Check sheet for the modelled part. Datum: model origin and axes. Units: mm. A direction names the side the tool comes from. Round coordinates to 2 decimals unless told otherwise and drop trailing zeros. Write each loop counter-clockwise with the first axis right and the second up, starting at its lowest first coordinate (ties: lowest second). Pieces come first, ordered by that corner, then holes.
from build123d import *

# Parameters (mm, degrees)
SKETCH1_W           = 60
SKETCH1_H           = 40
BOSS_EXTRUDE1_DEPTH = 4
CHAMFER1_SIZE       = 3
SKETCH2_W           = 36
SKETCH2_H           = 24
CUT_EXTRUDE1_DEPTH  = 1.5
SKETCH3_W           = 4
SKETCH3_H           = 24
BOSS_EXTRUDE2_DEPTH = 23
CHAMFER2_SIZE       = 3
CHAMFER3_SIZE       = 2
CHAMFER4_SIZE       = 2
CHAMFER5_SIZE       = 2
CUT_EXTRUDE2_DEPTH  = 2.5
SKETCH7_R           = 2.604037506
CUT_EXTRUDE3_DEPTH  = 70.285640648
CUT_EXTRUDE4_DEPTH  = 2.5
SKETCH12_R          = 2.604037506
CUT_EXTRUDE6_DEPTH  = 68.485183559


with BuildPart() as part:
    # Sketch1 → Boss-Extrude1 (new body)
    with BuildSketch(Plane(origin=(0, 0, 0), x_dir=(1, 0, 0), z_dir=(0, 1, 0))):
        with Locations((30, -20)):
            Rectangle(SKETCH1_W, SKETCH1_H)
    extrude(amount=BOSS_EXTRUDE1_DEPTH)

    # Chamfer1
    chamfer1_edges = [part.edges().sort_by_distance(p)[0] for p in [
        (0, 2, 0),
        (60, 2, 0),
        (60, 2, 40),
        (0, 2, 40),
    ]]
    chamfer(chamfer1_edges, length=CHAMFER1_SIZE)

    # Sketch2 → Cut-Extrude1 (cut)
    with BuildSketch(Plane(origin=(0, 4, 0), x_dir=(1, 0, 0), z_dir=(0, 1, 0))):
        with Locations((30, -12)):
            Rectangle(SKETCH2_W, SKETCH2_H)
    extrude(amount=-CUT_EXTRUDE1_DEPTH, mode=Mode.SUBTRACT)

    # Sketch3 → Boss-Extrude2 (add)
    with BuildSketch(Plane(origin=(0, 2.5, 0), x_dir=(1, 0, 0), z_dir=(0, 1, 0))):
        with Locations((50, -12)):
            Rectangle(SKETCH3_W, SKETCH3_H)
        with Locations((10, -12)):
            Rectangle(SKETCH3_W, SKETCH3_H)
    extrude(amount=BOSS_EXTRUDE2_DEPTH)

    # Chamfer2
    chamfer2_edges = [part.edges().sort_by_distance(p)[0] for p in [
        (50, 25.5, 24),
        (50, 25.5, 0),
        (10, 25.5, 0),
        (10, 25.5, 24),
    ]]
    chamfer(chamfer2_edges, length=CHAMFER2_SIZE)

    # Chamfer3
    chamfer3_edges = [part.edges().sort_by_distance(p)[0] for p in [
        (50, 4, 24),
        (10, 4, 24),
    ]]
    chamfer(chamfer3_edges, length=CHAMFER3_SIZE)

    # Chamfer4
    # the kernel refuses this chamfer: 2 mm, written as the material it takes off along each edge
    with BuildSketch(Plane(origin=(48, 4, 24), x_dir=(0, -0.9996219169112968, -0.027495876610585623), z_dir=(-1, 0, 0))) as chamfer4_piece_1_section:
        Polygon((CHAMFER4_SIZE * 0.999621916911, CHAMFER4_SIZE * 0.0274958766106), (-CHAMFER4_SIZE * 0.0274958766106, CHAMFER4_SIZE * 0.999621916911), (0, 0), align=None)
    chamfer4_piece_1 = extrude(amount=36, mode=Mode.PRIVATE)
    chamfer4_piece_1 = split(chamfer4_piece_1, bisect_by=Plane(origin=(30, 2.5, 24.699033576), z_dir=(0, 1, 0)), keep=Keep.TOP, mode=Mode.PRIVATE)
    chamfer4_piece_1 = split(chamfer4_piece_1, bisect_by=Plane(origin=(30, 4.361799404, 25.638200596), z_dir=(0, -0.7071067811865476, -0.7071067811865476)), keep=Keep.TOP, mode=Mode.PRIVATE)
    add(chamfer4_piece_1, mode=Mode.SUBTRACT)

    # Chamfer5
    # the kernel refuses this chamfer: 2 mm, written as the material it adds along each edge
    with BuildSketch(Plane(origin=(12, 2.5, 29.643365976), x_dir=(-0.027495876610586487, 0.9996219169112968, 0), z_dir=(0, 0, -1))) as chamfer5_piece_1_section:
        Polygon((CHAMFER5_SIZE * 0.999621916911, CHAMFER5_SIZE * 0.0274958766106), (-CHAMFER5_SIZE * 0.0274958766106, CHAMFER5_SIZE * 0.999621916911), (0, 0), align=None)
    chamfer5_piece_1 = extrude(amount=29.643365976, mode=Mode.PRIVATE)
    chamfer5_piece_1 = split(chamfer5_piece_1, bisect_by=Plane(origin=(12.696713147, 10.276643426, 19.723356574), z_dir=(0, -0.7071067811865476, -0.7071067811865476)), keep=Keep.TOP, mode=Mode.PRIVATE)
    add(chamfer5_piece_1)
    with BuildSketch(Plane(origin=(48, 2.5, 29.643365976), x_dir=(-0.9996219169112968, -0.027495876610586296, 0), z_dir=(0, 0, -1))) as chamfer5_piece_2_section:
        Polygon((CHAMFER5_SIZE * 0.999621916911, CHAMFER5_SIZE * 0.0274958766106), (-CHAMFER5_SIZE * 0.0274958766106, CHAMFER5_SIZE * 0.999621916911), (0, 0), align=None)
    chamfer5_piece_2 = extrude(amount=29.643365976, mode=Mode.PRIVATE)
    chamfer5_piece_2 = split(chamfer5_piece_2, bisect_by=Plane(origin=(47.833064516, 10.624596774, 19.375403226), z_dir=(0, -0.7071067811865476, -0.7071067811865476)), keep=Keep.TOP, mode=Mode.PRIVATE)
    add(chamfer5_piece_2)

    # Sketch4 → Cut-Extrude2 (cut)
    with BuildSketch(Plane.ZY.offset(-48)):
        Polygon((9.05620064, 16.5), (10.815025537, 25.5), (13.420692052, 25.5), (15.179516949, 16.5), (13.420692052, 4), (10.815025537, 4), align=None)
    extrude(amount=-CUT_EXTRUDE2_DEPTH, mode=Mode.SUBTRACT)

    # Sketch7 → Cut-Extrude3 (cut, through all)
    with BuildSketch(Plane.ZY.offset(-50.5)):
        with Locations((12.117858795, 16.5)):
            Circle(SKETCH7_R)
    extrude(amount=-CUT_EXTRUDE3_DEPTH, mode=Mode.SUBTRACT)

    # Sketch11 → Cut-Extrude4 (cut)
    with BuildSketch(Plane.ZY.offset(-12)):
        Polygon((9.05620064, 16.5), (10.815025537, 25.5), (13.420692052, 25.5), (15.179516949, 16.5), (13.420692052, 4), (10.815025537, 4), align=None)
    extrude(amount=CUT_EXTRUDE4_DEPTH, mode=Mode.SUBTRACT)

    # Sketch12 → Cut-Extrude6 (cut, through all)
    with BuildSketch(Plane.ZY.offset(-12)):
        with Locations((12.117858795, 16.5)):
            Circle(SKETCH12_R)
    extrude(amount=CUT_EXTRUDE6_DEPTH, mode=Mode.SUBTRACT)


solid = part.part
1. Go/stop test with flat-tipped pins: pin 1 (1.5 mm diameter, centred on x = 9, z = 26, fed in from +Y); pin 2 (3.5 mm diameter, centred on y = 18, z = 20.5, fed in from -X); pin 3 (1.8 mm diameter, centred on y = 19.5, z = 12.5, fed in from +X); pin 4 (3 mm diameter, centred on y = 16.5, z = 12.12, fed in from -X). Record where each tip stops, or that it passes through.
2. Sectioned sample at A-A, the plane z = 20. Enter the section's corners in (x, y).
3. Sectioned sample at D-D, the plane z = 38. Enter the section's corners in (x, y), plus the area to 3 significant figures.
4. Sectioned sample at B-B, the plane x = 35.5. Enter the section's corners in (y, z).
5. Set-up check for faces 5 (the flat face through (48, 15, 20)), 6 (the flat face through (9.5, 13, 12)), 7 (the flat face through (52, 12, 13)), 8 (the flat face through (47, 3.5, 13.2)): record each of +Z, -Z, +X, -X, +Y, -Y from which the full face is reachable in a straight line by a thin tool's end or side.
6. Scan lines: line 1 along X through (y, z) = (23.75, 12); line 2 along Z through (x, y) = (8.65, 16.5); line 3 along Y through (x, z) = (52, 26). Record each from-to range of solid material in increasing order.
7. Release check for a two-part mould opening along X. For faces 1 (the flat face through (13, 3.5, 13.2)), 2 (the flat face through (0, 2, 20)), 3 (the flat face through (59, 2, 38)), 4 (the flat face through (30, 0, 20)) record: released by +X, released by -X, zero draft, split by the parting line, or undercut.
8. Sectioned sample at C-C, the plane z = 30.5. Enter the section's corners in (x, y).
Computed values:
1. pin 1: stops at y = 4.75
1. pin 2: stops at x = 8
1. pin 3: stops at x = 52
1. pin 4: passes through
2. outline: (0, 0) - (60, 0) - (60, 4) - (52, 4) - (52, 25.5) - (48, 25.5) - (48, 4.5) - (46, 2.5) - (14, 2.5) - (12, 4.5) - (12, 25.5) - (8, 25.5) - (8, 4) - (0, 4) - close
3. outline: (1, 0) - (59, 0) - (59, 4) - (1, 4) - close
3. area: 232 mm2
4. outline: (0, 0) - (2.5, 0) - (2.5, 24.5) - (4, 26) - (4, 40) - (0, 40) - close
5. face 5: +Z, -Z, +Y
5. face 6: none
5. face 7: +Z, -Z, +X, +Y
5. face 8: -Z, +Y
6. line 1: x = 8 to 9.5, 50.5 to 52
6. line 2: z = 0 to 9.51, 14.72 to 24
6. line 3: y = 0 to 4
7. face 1: undercut
7. face 2: released by -X
7. face 3: released by +X
7. face 4: zero draft
8. outline: (0, 0) - (60, 0) - (60, 4) - (0, 4) - close
